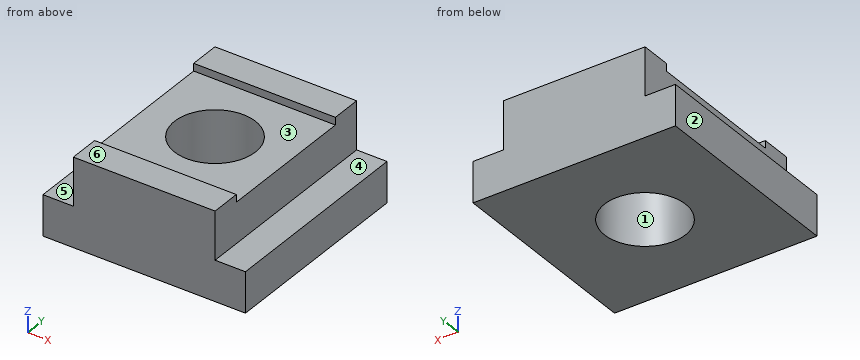
from build123d import *

# Parameters (mm, degrees)
F0_W     = 70
F0_H     = 23.720817
F2_DEPTH = 1000
F1_W     = 100
F1_H     = 100
F1_W_2   = 70
F1_H_2   = 70
F3_DEPTH = 1000
F1_R     = 20
F4_DEPTH = 40


with BuildPart() as f2:
    # F0 (on Front) → F2 (new body)
    with BuildSketch(Plane.XZ):
        Polygon((0, 20), (0, 0), (100, 0), (100, 20), (85, 20), (15, 20), align=None)
        with Locations((50, 31.860408)):
            Rectangle(F0_W, F0_H)
    extrude(amount=-F2_DEPTH)

    # F1 (on Top) → F3 (intersect)
    with BuildSketch(Plane.XY):
        with Locations((50, 50)):
            Rectangle(F1_W, F1_H)
        with Locations((50, 50)):
            Rectangle(F1_W_2, F1_H_2, mode=Mode.SUBTRACT)
    extrude(amount=F3_DEPTH, mode=Mode.INTERSECT)

    # F1 (on Top) → F4 (join)
    with BuildSketch(Plane.XY):
        with Locations((50, 50)):
            Rectangle(F1_W_2, F1_H_2)
        with Locations((50, 50)):
            Circle(F1_R, mode=Mode.SUBTRACT)
    extrude(amount=F4_DEPTH)


solid = f2.part
For this review, take the finished solid that the model builds, in its own axes (mm). Face numbers are marked on the shaded views. A direction names the side the tool comes from. Give positions to 0.01 mm unless a question says otherwise; leave off trailing zeros. Loops run counter-clockwise (first coordinate to the right, second up) from the corner with the lowest first, then second, coordinate; pieces in that order, holes last. Notation, with made-up numbers: (77.25, 14) - (130.25, 14) arc R24 ccw to (130.25, 27) - close; hole circle Ø3 at (79, -38.5). An arc over 180 degrees is marked (long way). Write each question's results on one line, items separated by ' | '.
(1) Take a section at A-A (x = 50). Give the boundary of the cut face in (y, z), then the cut area to 3 significant figures.
Conclusion:
outline: (0, 0) - (30, 0) - (30, 40) - (15, 40) - (15, 43.72) - (0, 43.72) - close; (70, 0) - (100, 0) - (100, 43.72) - (85, 43.72) - (85, 40) - (70, 40) - close | area: 2,510 mm^2
(2) Take a section at B-B (y = 50). Give the boundary of the cut face in (x, z), then the cut area to 3 significant figures.
Conclusion:
outline: (0, 0) - (30, 0) - (30, 40) - (15, 40) - (15, 20) - (0, 20) - close; (70, 0) - (100, 0) - (100, 20) - (85, 20) - (85, 40) - (70, 40) - close | area: 1,800 mm^2
(3) For the marked faces 4, 5 and 6, list the 3-axis set-ups (+Z, -Z, +X, -X, +Y, -Y) from which the entire face can be reached by the end or side of a thin tool; tool diameter is ignored.
Conclusion:
face 4: +Z, +X, +Y, -Y | face 5: +Z, -X, +Y, -Y | face 6: +Z, +X, -X, +Y, -Y
(4) Draft analysis for pull direction X (two halves, no side actions). For the marked faces 1, 2 and 3, state which applies: +X half, -X half, draft (parallel to the pull), parting line (faces both ways), or undercut.
Conclusion:
face 1: undercut | face 2: -X half | face 3: draft
(5) Take a section at C-C (z = 18.5). Give the boundary of the cut face in (x, y).
Conclusion:
outline: (0, 0) - (100, 0) - (100, 100) - (0, 100) - close; hole circle Ø40 at (50, 50)
(6) Take a section at D-D (x = 22). Give the boundary of the cut face in (y, z), then the cut area to 3 significant figures.
Conclusion:
outline: (0, 0) - (100, 0) - (100, 43.72) - (85, 43.72) - (85, 40) - (15, 40) - (15, 43.72) - (0, 43.72) - close | area: 4,110 mm^2
(7) For line 1 along Y through (x, z) = (50, 27); line 2 along Y through (x, z) = (46, 41); line 3 along Z through (x, y) = (80, 45), list the stretches that pass through material, from the lowest coordinate up.
Conclusion:
line 1: 0 to 30, 70 to 100 | line 2: 0 to 15, 85 to 100 | line 3: 0 to 40
(8) For pin 1 Ø12 at (x, y) = (6, 51) entering from +Z; pin 2 Ø19 at (y, z) = (69.5, 30.5) entering from -X; pin 3 Ø12 at (y, z) = (76.5, 30) entering from +X, all flat-tipped, find the tip position at first contact; note any pin that passes through.
Conclusion:
pin 1: z = 20 | pin 2: x = 15 | pin 3: x = 85
